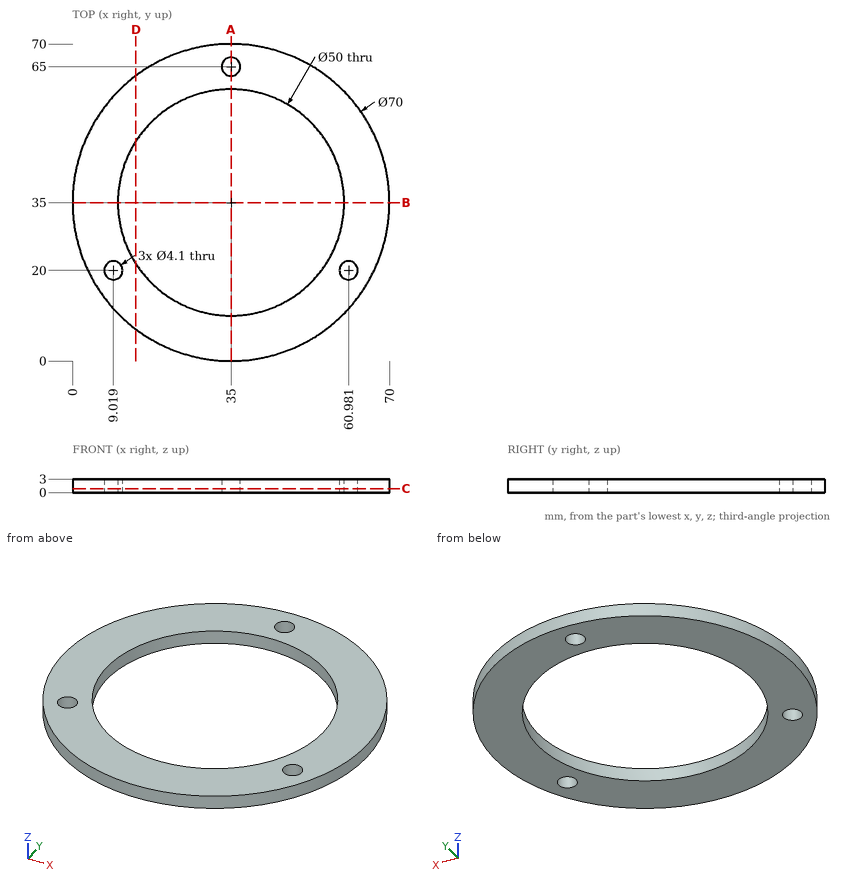
Print and shaded views of the part. All mm, measured from the part's lowest x, y and z. Give positions to 0.01 mm unless a question says otherwise; leave off trailing zeros. Loops run counter-clockwise (first coordinate to the right, second up) from the corner with the lowest first, then second, coordinate; pieces in that order, holes last. Notation, with made-up numbers: (78, 58) -> (109, 58) arc R12 ccw to (109, 78) -> close; hole circle Ø6 at (-5.75, -5.75). An arc over 180 degrees is marked (long way). One line per question, with ' | ' between items. Start each with the question number.
1) Probe L1, parallel to Y at x = 35, z = 2.1; L2, parallel to Y at x = 46.5, z = 1.1; L3, parallel to Y at x = 30, z = 2.5. List the from-to ranges inside material, lowest first.
2) Cut at B-B (y = 35). Give the cut face in (x, z).
3) Cut at C-C (z = 0.9). Give the cut face in (x, y), plus the area to 3 significant figures.
4) Cut at A-A (x = 35). Give the cut face in (y, z), plus the area to 3 significant figures.
5) Cut at D-D (x = 14). Give the cut face in (y, z).
6) Pin check, flat tips, straight feed: pin 1 (5.5 mm diameter, centred on x = 60.981, y = 20, fed in from -Z); pin 2 (1.5 mm diameter, centred on y = 26, z = 1.5, fed in from -X); pin 3 (1.5 mm diameter, centred on x = 10.5, z = 2.5, fed in from +Y). Stop position of each tip, or through.
Return value:
1) L1: 0 to 10, 60 to 62.95, 67.05 to 70 | L2: 1.94 to 12.8, 57.2 to 68.06 | L3: 0.36 to 10.51, 59.49 to 69.64
2) outline: (0, 0) -> (10, 0) -> (10, 3) -> (0, 3) -> close; (60, 0) -> (70, 0) -> (70, 3) -> (60, 3) -> close
3) outline: circle Ø70 at (35, 35); hole circle Ø4.1 at (9.02, 20); hole circle Ø50 at (35, 35); hole circle Ø4.1 at (35, 65); hole circle Ø4.1 at (60.98, 20) | area: 1,850 mm^2
4) outline: (0, 0) -> (10, 0) -> (10, 3) -> (0, 3) -> close; (60, 0) -> (62.95, 0) -> (62.95, 3) -> (60, 3) -> close; (67.05, 0) -> (70, 0) -> (70, 3) -> (67.05, 3) -> close | area: 47.7 mm^2
5) outline: (7, 0) -> (21.44, 0) -> (21.44, 3) -> (7, 3) -> close; (48.56, 0) -> (63, 0) -> (63, 3) -> (48.56, 3) -> close
6) pin 1: z = 0 | pin 2: x = 0.99 | pin 3: y = 60.71
